from build123d import *

# Parameters (mm, degrees)
BACKSKETCH_W        = 38.1
BACKSKETCH_H        = 50.8
BACKSKETCH_R        = 1.4732
BACKSKETCH_R_2      = 3.429
BOSS_EXTRUDE1_DEPTH = 3.0734


with BuildPart() as part:
    # backSketch → Boss-Extrude1 (new body)
    # profile 1 of 3: a face of its own
    with BuildSketch(Plane.XY):
        Polygon((19.05, 0), (0, 0), (0, 25.4), (-3.0734, 25.4), (-3.0734, -3.0734), (19.05, -3.0734), align=None)
    # profile 2 of 3: a face of its own
    with BuildSketch(Plane.XY):
        with Locations((19.05, 25.4)):
            Rectangle(BACKSKETCH_W, BACKSKETCH_H)
        with Locations((19.196716748, 36.578509469)):
            Circle(BACKSKETCH_R, mode=Mode.SUBTRACT)
        with Locations((13.465150567, 18.677705992)):
            Circle(BACKSKETCH_R_2, mode=Mode.SUBTRACT)
    # profile 3 of 3: a face of its own
    with BuildSketch(Plane.XY):
        Polygon((38.1, 50.8), (38.1, 25.4), (41.1734, 25.4), (41.1734, 53.8734), (19.196716748, 53.8734), (19.196716748, 50.8), align=None)
    extrude(amount=BOSS_EXTRUDE1_DEPTH)


solid = part.part
Can you work these out from the model? Positions are in its coordinate system, mm. A direction names the side the tool comes from. Round coordinates to 2 decimals unless told otherwise and drop trailing zeros. Loops run counter-clockwise (first coordinate to the right, second up) from the corner with the lowest first, then second, coordinate; pieces in that order, holes last. Notation, with made-up numbers: (77.25, -30.5) - (99.25, -30.5) arc R30 cw to (99.25, -0.5) - close; hole circle Ø9 at (39.5, 4.25). An arc over 180 degrees is marked (long way). Answer in a Markdown table with one row per item. Add a question column.
Q1. For pin 1 Ø0.9 at (y, z) = (-2, 1) entering from +X; pin 2 Ø0.9 at (y, z) = (36, 2) entering from -X; pin 3 Ø1.5 at (x, z) = (30.5, 2.5) entering from -Y, each with a flat end and sliding along its axis, tell me the tip position at first contact or that it passes through.
Q2. I want a section at D-D on y = 14. List the corners of the cut face in (x, z) for me.
Q3. We'd pull the mould along Y, two halves only. Please class faces 4 (the flat face through (19.197, 52, 2)), 5 (the flat face through (40, 25.4, 2)), 6 (the cylindrical face through (10.94, 21, 1.52)): pulls with the +Y half, pulls with the -Y half, needs draft (parallel to the pull), parting line crosses it, or undercut.
Q4. I need wall thicknesses on L1, parallel to X at y = 9.5, z = 1.35; L2, parallel to X at y = 44, z = 1.9; L3, parallel to Y at x = 0.5, z = 0.9. Which ranges of each line are inside material? Lowest first, please.
Q5. I want a section at A-A on z = 2.05. List the corners of the cut face in (x, y) for me, and give its area (3 significant figures).
Q6. I want a section at C-C on x = 9. List the corners of the cut face in (y, z) for me, and give its area (3 significant figures).
Q7. I want a section at B-B on y = 20. List the corners of the cut face in (x, z) for me, and give its area (3 significant figures).
Q8. Which directions (+Z, -Z, +X, -X, +Y, -Y) give clear straight access to the entire face, cutting with the end or side of a thin tool? Please do faces 1 (the flat face through (9, 50.8, 2)), 2 (the flat face through (8, -3.073, 2)), 3 (the flat face through (19.05, -2, 2)).
A:
| question | item | result |
|---|---|---|
| 1 | pin 1 | x = 19.05 |
| 1 | pin 2 | x = 0 |
| 1 | pin 3 | y = 0 |
| 2 | outline | (-3.07, 0) - (38.1, 0) - (38.1, 3.07) - (-3.07, 3.07) - close |
| 3 | face 4 | needs draft |
| 3 | face 5 | pulls with the -Y half |
| 3 | face 6 | undercut |
| 4 | L1 | -3.07 to 38.1 |
| 4 | L2 | 0 to 41.17 |
| 4 | L3 | -3.07 to 50.8 |
| 5 | outline | (-3.07, -3.07) - (19.05, -3.07) - (19.05, 0) - (38.1, 0) - (38.1, 25.4) - (41.17, 25.4) - (41.17, 53.87) - (19.2, 53.87) - (19.2, 50.8) - (0, 50.8) - (0, 25.4) - (-3.07, 25.4) - close; hole circle Ø6.86 at (13.47, 18.68); hole circle Ø2.95 at (19.2, 36.58) |
| 5 | area | 2,180 mm^2 |
| 6 | outline | (-3.07, 0) - (50.8, 0) - (50.8, 3.07) - (-3.07, 3.07) - close |
| 6 | area | 166 mm^2 |
| 7 | outline | (-3.07, 0) - (10.3, 0) - (10.3, 3.07) - (-3.07, 3.07) - close; (16.63, 0) - (38.1, 0) - (38.1, 3.07) - (16.63, 3.07) - close |
| 7 | area | 107 mm^2 |
| 8 | face 1 | +Z, -Z, -X, +Y |
| 8 | face 2 | +Z, -Z, +X, -X, -Y |
| 8 | face 3 | +Z, -Z, +X, -Y |
